from build123d import *

# Parameters (mm, degrees)
SKETCH_1_W          = 100
SKETCH_1_H          = 35
EXTRUDE_1_DEPTH     = 15
SKETCH_2_W          = 100
SKETCH_2_H          = 60
EXTRUDE_2_DEPTH     = 15
SKETCH_3_R          = 3.5
CUT_EXTRUDE_1_DEPTH = 113.388833965
SKETCH_4_R          = 5.5
CUT_EXTRUDE_2_DEPTH = 7
SKETCH_5_R          = 4.5
SKETCH_5_R_2        = 8
CUT_EXTRUDE_3_DEPTH = 113.388833965
SKETCH_6_R          = 12
CUT_EXTRUDE_4_DEPTH = 8
SKETCH_7_R          = 6.5
CUT_EXTRUDE_5_DEPTH = 8


with BuildPart() as part:
    # 草图1 → 凸台-拉伸1 (new body)
    with BuildSketch(Plane.XY):
        with Locations((50, 17.5)):
            Rectangle(SKETCH_1_W, SKETCH_1_H)
    extrude(amount=EXTRUDE_1_DEPTH)

    # 草图2 → 凸台-拉伸2 (add)
    with BuildSketch(Plane.XZ):
        with Locations((50, 7.5)):
            Rectangle(SKETCH_2_W, SKETCH_2_H)
    extrude(amount=EXTRUDE_2_DEPTH)

    # 草图3 → 切除-拉伸1 (cut, through all)
    with BuildSketch(Plane(origin=(0, 0, 0), x_dir=(1, 0, 0), z_dir=(0, 1, 0))):
        with Locations(Location((10, 7.5, 0), (0, 0, 270))):
            Circle(SKETCH_3_R)
        with Locations(Location((90, 7.5, 0), (0, 0, 270))):
            Circle(SKETCH_3_R)
        with Locations(Location((90, -22.5, 0), (0, 0, 90))):
            Circle(SKETCH_3_R)
        with Locations(Location((10, -22.5, 0), (0, 0, 90))):
            Circle(SKETCH_3_R)
    extrude(amount=-CUT_EXTRUDE_1_DEPTH, mode=Mode.SUBTRACT)

    # 草图4 → 切除-拉伸2 (cut)
    with BuildSketch(Plane(origin=(0, 0, 0), x_dir=(1, 0, 0), z_dir=(0, 1, 0))):
        with Locations(Location((10, 7.5, 0), (0, 0, 270))):
            Circle(SKETCH_4_R)
        with Locations(Location((90, 7.5, 0), (0, 0, 270))):
            Circle(SKETCH_4_R)
        with Locations(Location((10, -22.5, 0), (0, 0, 270))):
            Circle(SKETCH_4_R)
        with Locations(Location((90, -22.5, 0), (0, 0, 270))):
            Circle(SKETCH_4_R)
    extrude(amount=-CUT_EXTRUDE_2_DEPTH, mode=Mode.SUBTRACT)

    # 草图5 → 切除-拉伸3 (cut, through all)
    with BuildSketch(Plane(origin=(0, 0, 0), x_dir=(-1, 0, 0), z_dir=(0, 0, -1))):
        with Locations((-85, 20)):
            Circle(SKETCH_5_R)
        with Locations((-15, 20)):
            Circle(SKETCH_5_R)
        with Locations((-50, 20)):
            Circle(SKETCH_5_R_2)
    extrude(amount=-CUT_EXTRUDE_3_DEPTH, mode=Mode.SUBTRACT)

    # 草图6 → 切除-拉伸4 (cut)
    with BuildSketch(Plane(origin=(0, 0, 0), x_dir=(-1, 0, 0), z_dir=(0, 0, -1))):
        with Locations((-50, 20)):
            Circle(SKETCH_6_R)
    extrude(amount=-CUT_EXTRUDE_4_DEPTH, mode=Mode.SUBTRACT)

    # 草图7 → 切除-拉伸5 (cut)
    with BuildSketch(Plane.XY.offset(15)):
        with Locations((15, 20)):
            Circle(SKETCH_7_R)
        with Locations((85, 20)):
            Circle(SKETCH_7_R)
    extrude(amount=-CUT_EXTRUDE_5_DEPTH, mode=Mode.SUBTRACT)


solid = part.part
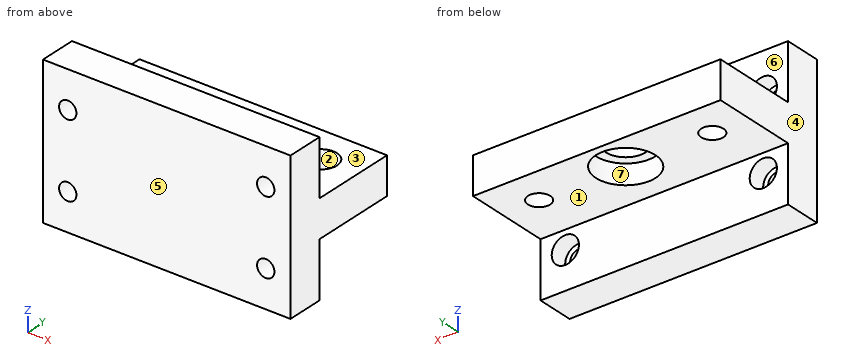
Work out the finished part from the listing and answer in its coordinate system (mm). Face numbers are marked on the shaded views. A direction names the side the tool comes from. Coordinates: 2 decimals unless noted, no trailing zeros. Loops run counter-clockwise (first coordinate to the right, second up) from the corner with the lowest first, then second, coordinate; pieces in that order, holes last. Notation, with made-up numbers: M 54.25,-35.5 L 65.25,-35.5 A23 ccw 65.25,-1.5 Z; hole C 83,-37 d4. An arc over 180 degrees is marked long. Answer in a Markdown table with one row per item. Add a question column.
1. Consider L1, parallel to X at y = -4, z = -7; L2, parallel to X at y = -11, z = -7.5; L3, parallel to Z at x = 89.5, y = 18. Determine where each line is inside the solid, lowest interval first.
2. Flat-ended cylindrical pins translate along their axes: P1, Ø21, axis at x = 85, y = 20, coming from the +Z side; P2, Ø12, axis at x = 10.5, z = 21.5, coming from the +Y side; P3, Ø10.5, axis at x = 85, y = 20, coming from the -Z side. Find the tip coordinate at first contact, or state that the pin passes through.
3. The mould has two halves that part along Y. Classify the marked faces 4, 5, 6 and 7: pulls with the +Y half, pulls with the -Y half, needs draft (parallel to the pull), parting line crosses it, or undercut.
4. Find section B-B, the plane z = 12.5. Write down the section's boundary in (x, y), then the cut area to 3 significant figures.
5. Find section A-A, the plane z = -7.5. Write down the section's boundary in (x, y).
6. Find section D-D, the plane y = 17.5. Write down the section's boundary in (x, z), then the cut area to 3 significant figures.
7. Find section C-C, the plane x = 68.5. Write down the section's boundary in (y, z).
8. A tool of negligible diameter and unlimited length cuts with its end or side. For the marked faces 1, 2 and 3, from which of +Z, -Z, +X, -X, +Y, -Y can it reach the whole face along a straight path? Write none if from no direction.
Reported:
| question | item | result |
|---|---|---|
| 1 | L1 | x = 0 to 4.52, 15.48 to 84.52, 95.48 to 100 |
| 1 | L2 | x = 0 to 6.5, 13.5 to 86.5, 93.5 to 100 |
| 1 | L3 | z = 0 to 7 |
| 2 | P1 | stops at z = 15 |
| 2 | P2 | stops at y = 0 |
| 2 | P3 | stops at z = 0 |
| 3 | face 4 | needs draft |
| 3 | face 5 | pulls with the -Y half |
| 3 | face 6 | pulls with the +Y half |
| 3 | face 7 | undercut |
| 4 | outline | M 0,-15 L 100,-15 L 100,35 L 0,35 Z; hole C 15,20 d13; hole C 50,20 d16; hole C 85,20 d13 |
| 4 | area | 4,530 mm^2 |
| 5 | outline | M 0,-15 L 6.5,-15 L 6.5,-7 L 4.5,-7 L 4.5,0 L 0,0 Z; M 13.5,-15 L 86.5,-15 L 86.5,-7 L 84.5,-7 L 84.5,0 L 15.5,0 L 15.5,-7 L 13.5,-7 Z; M 93.5,-15 L 100,-15 L 100,0 L 95.5,0 L 95.5,-7 L 93.5,-7 Z |
| 6 | outline | M 0,0 L 11.26,0 L 11.26,7 L 9,7 L 9,15 L 0,15 Z; M 18.74,0 L 38.26,0 L 38.26,8 L 42.4,8 L 42.4,15 L 21,15 L 21,7 L 18.74,7 Z; M 57.6,8 L 61.74,8 L 61.74,0 L 81.26,0 L 81.26,7 L 79,7 L 79,15 L 57.6,15 Z; M 88.74,0 L 100,0 L 100,15 L 91,15 L 91,7 L 88.74,7 Z |
| 6 | area | 909 mm^2 |
| 7 | outline | M -15,-22.5 L 0,-22.5 L 0,0 L 35,0 L 35,15 L 0,15 L 0,37.5 L -15,37.5 Z |
| 8 | face 1 | -Z, +X, -X, +Y |
| 8 | face 2 | +Z |
| 8 | face 3 | +Z, +X, -X, +Y |
